Work out the finished part from the listing and answer in its coordinate system (mm). A direction names the side the tool comes from. Coordinates: 2 decimals unless noted, no trailing zeros. Order: outer loops, then holes, each group sorted by start corner. A loop starts at its lowest first (then second) coordinate and runs counter-clockwise, first axis right, second up. Notation, with made-up numbers: M 13,37 L 60,37 A16 cw 60,55 Z; hole C 38,-28 d1. An arc over 180 degrees is marked long. Write item = value, one per line. Start each with the question number.
Q1. Find section B-B on z = 11. Give the vertices of the cut face in (x, y).
Q2. Find section D-D on z = 21.5. Give the vertices of the cut face in (x, y).
Q3. Straight lines are drawn through the part: line 1 along X through (y, z) = (2, 37); line 2 along X through (y, z) = (4.25, 8.5); line 3 along Z through (x, y) = (35.5, 5.5). For each, find the intervals that lie inside material, in ascending order.
Q4. Each of these flat-tipped pins is pushed along its axis until it touches: P1, Ø3, axis at x = -2.5, y = 3, coming from the -Z side; P2, Ø4, axis at x = 57, y = 3, coming from the +Z side; P3, Ø12, axis at x = 28, z = 28, coming from the +Y side. Where does it stop, or does it pass through?
Q5. Determine the mould class of faces 1 (the cylindrical face through (5.295, 0.591, 7.205)), 2 (the flat face through (7, 3.81, 4)), 3 (the flat face through (57, 11.43, 21)) for opening direction Y: released by +Y, released by -Y, zero draft, split by the parting line, or undercut.
Q6. Find section C-C on y = 6.25. Give the vertices of the cut face in (x, z).
Q7. A tool of negligible diameter and unlimited length cuts with its end or side. For faces 4 (the conical face through (56.576, 18.688, 43.811)), 5 (the cylindrical face through (1.45, 9.66, 40.64)), 6 (the flat face through (-2, 11.43, 21)), from which of +Z, -Z, +X, -X, +Y, -Y can it reach the whole face along a straight path? Write none if from no direction.
Q8. Find section A-A on y = 15.5. Give the vertices of the cut face in (x, z), and give its area (3 significant figures).
```python
from build123d import *

# Parameters (mm, degrees)
SKETCH1_W                    = 62.484
SKETCH1_H                    = 49.784
SKETCH1_W_2                  = 54.864
SKETCH1_H_2                  = 42.164
BOSS_EXTRUDE1_DEPTH          = 19.05
SKETCH3_W                    = 62.484
SKETCH3_H                    = 49.784
BOSS_EXTRUDE2_DEPTH          = 3.81
FILLET1_R                    = 5.08
SKETCH4_R                    = 3.81
BOSS_EXTRUDE3_DEPTH          = 3.81
F_4_0_4_DIAMETER_HOLE1_D     = 4
F_4_0_4_DIAMETER_HOLE1_DEPTH = 6.35
F_4_0_4_DIAMETER_HOLE1_TIP   = 1.201721238
CUT_EXTRUDE1_REACH           = 81.88
SKETCH8_W                    = 21.59
SKETCH8_H                    = 11.43
CUT_EXTRUDE2_REACH           = 81.88
SKETCH9_W                    = 16.002
SKETCH9_H                    = 11.43
FILLET2_R                    = 5.08
CHAMFER1_SIZE                = 1.27
CHAMFER2_SIZE                = 0.508


with BuildPart() as part:
    # Sketch1 → Boss-Extrude1 (new body)
    with BuildSketch(Plane(origin=(0, 0, 0), x_dir=(1, 0, 0), z_dir=(0, 1, 0))):
        with Locations((27.432, -21.082)):
            Rectangle(SKETCH1_W, SKETCH1_H)
        with Locations((27.432, -21.082)):
            Rectangle(SKETCH1_W_2, SKETCH1_H_2, mode=Mode.SUBTRACT)
    extrude(amount=BOSS_EXTRUDE1_DEPTH)

    # Sketch3 → Boss-Extrude2 (add)
    with BuildSketch(Plane.XZ):
        with Locations((27.432, 21.082)):
            Rectangle(SKETCH3_W, SKETCH3_H)
    extrude(amount=BOSS_EXTRUDE2_DEPTH)

    # Fillet1
    fillet1_edges = [part.edges().sort_by_distance(p)[0] for p in [
        (0, 9.525, 0),
        (0, 9.525, 42.164),
        (54.864, 9.525, 42.164),
        (54.864, 9.525, 0),
    ]]
    fillet(fillet1_edges, radius=FILLET1_R)

    # Sketch4 → Boss-Extrude3 (add)
    with BuildSketch(Plane(origin=(0, 0, 0), x_dir=(1, 0, 0), z_dir=(0, 1, 0))):
        with Locations(Location((49.657, -5.207, 0), (0, 0, 90))):
            Circle(SKETCH4_R)
        with Locations(Location((49.657, -36.957, 0), (0, 0, 90))):
            Circle(SKETCH4_R)
        with Locations(Location((5.207, -36.957, 0), (0, 0, 90))):
            Circle(SKETCH4_R)
        with Locations(Location((5.207, -5.207, 0), (0, 0, 90))):
            Circle(SKETCH4_R)
    extrude(amount=BOSS_EXTRUDE3_DEPTH)

    # Ø4.0 (4) Diameter Hole1
    with Locations(Plane(origin=(5.207, 3.81, 5.207), x_dir=(0, 0, 1), z_dir=(0, 1, 0))):
        with Locations((0, 0), (31.75, 0), (31.75, 44.45), (0, 44.45)):
            Hole(F_4_0_4_DIAMETER_HOLE1_D / 2, depth=F_4_0_4_DIAMETER_HOLE1_DEPTH)
            with Locations((0, 0, -(F_4_0_4_DIAMETER_HOLE1_DEPTH + F_4_0_4_DIAMETER_HOLE1_TIP / 2))):  # 118° drill point
                Cone(0, F_4_0_4_DIAMETER_HOLE1_D / 2, F_4_0_4_DIAMETER_HOLE1_TIP, mode=Mode.SUBTRACT)

    # Sketch8 → Cut-Extrude1 (cut, up to next)
    with BuildSketch(Plane(origin=(58.674, 0, 0), x_dir=(0, 0, -1), z_dir=(1, 0, 0)), mode=Mode.PRIVATE) as cut_extrude1_sk1:
        with Locations((-21.082, 5.715)):
            Rectangle(SKETCH8_W, SKETCH8_H)
    cut_extrude1_tool1 = extrude(cut_extrude1_sk1.sketch, amount=-CUT_EXTRUDE1_REACH, mode=Mode.PRIVATE) & part.part
    add(cut_extrude1_tool1.solids().sort_by_distance((58.674, 5.715, 21.082))[0], mode=Mode.SUBTRACT)

    # Sketch9 → Cut-Extrude2 (cut, up to next)
    with BuildSketch(Plane.ZY.offset(3.81), mode=Mode.PRIVATE) as cut_extrude2_sk1:
        with Locations((21.082, 5.715)):
            Rectangle(SKETCH9_W, SKETCH9_H)
    cut_extrude2_tool1 = extrude(cut_extrude2_sk1.sketch, amount=-CUT_EXTRUDE2_REACH, mode=Mode.PRIVATE) & part.part
    add(cut_extrude2_tool1.solids().sort_by_distance((-3.81, 5.715, 21.082))[0], mode=Mode.SUBTRACT)

    # Fillet2
    fillet2_edges = [part.edges().sort_by_distance(p)[0] for p in [
        (-3.81, 7.62, -3.81),
        (58.674, 7.62, -3.81),
        (58.674, 7.62, 45.974),
        (-3.81, 7.62, 45.974),
    ]]
    fillet(fillet2_edges, radius=FILLET2_R)

    # Chamfer1
    chamfer1_edges = [part.edges().sort_by_distance(p)[0] for p in [
        (-3.81, 19.05, 21.082),
        (27.432, 19.05, -3.81),
        (27.432, 19.05, 45.974),
        (58.674, 19.05, 21.082),
        (-2.322102448, 19.05, 44.486102448),
        (57.186102448, 19.05, 44.486102448),
        (57.186102448, 19.05, -2.322102448),
        (-2.322102448, 19.05, -2.322102448),
    ]]
    chamfer(chamfer1_edges, length=CHAMFER1_SIZE)

    # Chamfer2
    chamfer2_edges = [part.edges().sort_by_distance(p)[0] for p in [
        (49.657, 3.81, 9.017),
        (49.657, 3.81, 40.767),
        (5.207, 3.81, 40.767),
        (5.207, 3.81, 9.017),
    ]]
    chamfer(chamfer2_edges, length=CHAMFER2_SIZE)


solid = part.part
```
Findings below:
q1.outline = M -3.81,-3.81 L 58.67,-3.81 L 58.67,0 L 0,0 L 0,19.05 L -2.54,19.05 L -3.81,17.78 Z; M 54.86,11.43 L 58.67,11.43 L 58.67,17.78 L 57.4,19.05 L 54.86,19.05 Z
q2.outline = M -3.81,-3.81 L 58.67,-3.81 L 58.67,0 L -3.81,0 Z; M -3.81,11.43 L 0,11.43 L 0,19.05 L -2.54,19.05 L -3.81,17.78 Z; M 54.86,11.43 L 58.67,11.43 L 58.67,17.78 L 57.4,19.05 L 54.86,19.05 Z
q3.line_1 = -3.81 to 0, 1.4 to 3.21, 7.21 to 9.02, 45.85 to 47.66, 51.66 to 53.47, 54.86 to 58.67
q3.line_2 = -3.81 to 0, 54.86 to 58.67
q3.line_3 = -3.81 to 0, 42.16 to 45.97
q4.P1 = -3.27
q4.P2 = 45.78
q4.P3 = 0
q5.face_1 = zero draft
q5.face_2 = released by +Y
q5.face_3 = undercut
q6.outline = M -3.81,1.27 A5.08 ccw 1.27,-3.81 L 53.59,-3.81 A5.08 ccw 58.67,1.27 L 58.67,10.29 L 54.86,10.29 L 54.86,5.08 A5.08 cw 49.78,0 L 5.08,0 A5.08 cw 0,5.08 L 0,13.08 L -3.81,13.08 Z; M -3.81,29.08 L 0,29.08 L 0,37.08 A5.08 cw 5.08,42.16 L 49.78,42.16 A5.08 cw 54.86,37.08 L 54.86,31.88 L 58.67,31.88 L 58.67,40.89 A5.08 ccw 53.59,45.97 L 1.27,45.97 A5.08 ccw -3.81,40.89 Z
q7.face_4 = +Z, +X, +Y
q7.face_5 = +Y
q7.face_6 = +X, -X
q8.outline = M -3.81,1.27 A5.08 ccw 1.27,-3.81 L 53.59,-3.81 A5.08 ccw 58.67,1.27 L 58.67,40.89 A5.08 ccw 53.59,45.97 L 1.27,45.97 A5.08 ccw -3.81,40.89 Z; hole M 0,5.08 A5.08 ccw 5.08,0 L 49.78,0 A5.08 ccw 54.86,5.08 L 54.86,37.08 A5.08 ccw 49.78,42.16 L 5.08,42.16 A5.08 ccw 0,37.08 Z
q8.area = 797 mm^2
